Autodesk Inventor part; units mm, degrees
ref_plane "YZ Plane" through (0, 0, 0) normal (1, 0, 0) x (0, 1, 0)
ref_plane "XZ Plane" through (0, 0, 0) normal (0, 1, 0) x (-1, 0, 0)
ref_plane "XY Plane" through (0, 0, 0) normal (0, 0, 1) x (1, 0, 0)
sketch "Base" plane through (0, 0, 0) normal (0, 0, 1) x (1, 0, 0)
  line L0 (-22, -39.56) -> (22, -39.56)
  line L1 (22, -39.56) -> (22, 39.56)
  line L2 (22, 39.56) -> (-22, 39.56)
  line L3 (-22, 39.56) -> (-22, -39.56)
  line L4 (-22, -39.56) -> (22, 39.56) construction
  line L5 (22, -39.56) -> (-22, 39.56) construction
  point P0 (0, 0)
  dimension "d56" = 44
  dimension "d57" = 79.12
extrude "Extrusion4" add sketch "Base" along normal blind 6
sketch "Slot1" plane through (0, 0, 6) normal (0, 0, 1) x (1, 0, 0)
  line L0 (21, -38.56) -> (-21, -38.56)
  line L1 (-21, -38.56) -> (-21, -30.44)
  line L2 (-21, -30.44) -> (21, -30.44)
  line L3 (21, -30.44) -> (21, -38.56)
  line L4 (21, -38.56) -> (-21, -30.44) construction
  line L5 (-21, -38.56) -> (21, -30.44) construction
  line L6 (22, -39.56) -> (22, 39.56)
  line L7 (-22, -39.56) -> (22, -39.56)
  point P0 (0, 0)
  point P1 (0, -34.5)
  dimension "d62" = 8.12
  dimension "d63" = 1
  dimension "d64" = 42
  dimension "d66" = 1
extrude "Slot1 slot" cut sketch "Slot1" against normal blind 4
sketch "Slot2" plane through (0, 0, 6) normal (0, 0, 1) x (1, 0, 0)
  line L0 (21, -0.44) -> (-21, -0.44)
  line L1 (-21, -0.44) -> (-21, 6.08)
  line L2 (-21, 6.08) -> (21, 6.08)
  line L3 (21, 6.08) -> (21, -0.44)
  line L4 (21, -0.44) -> (-21, 6.08) construction
  line L5 (-21, -0.44) -> (21, 6.08) construction
  line L6 (-22, 39.56) -> (-22, -39.56)
  line L7 (-21, -30.44) -> (21, -30.44)
  point P0 (0, 0)
  point P1 (0, 2.82)
  dimension "d75" = 6.52
  dimension "d76" = 42
  dimension "d77" = 1
  dimension "d80" = 30
extrude "Slot2 slot" cut sketch "Slot2" against normal blind 4
sketch "Slot3" plane through (0, 0, 6) normal (0, 0, 1) x (1, 0, 0)
  line L0 (-21, 38.2) -> (21, 38.2)
  line L1 (21, 38.2) -> (21, 34.08)
  line L2 (21, 34.08) -> (-21, 34.08)
  line L3 (-21, 34.08) -> (-21, 38.2)
  line L4 (-21, 38.2) -> (21, 34.08) construction
  line L5 (21, 38.2) -> (-21, 34.08) construction
  point P0 (0, 36.14)
  dimension "d83" = 4.12
  dimension "d84" = 42
extrude "Extrusion7" cut sketch "Slot3" against normal blind 4
fillet "Fillet1" radius 2 1 edges at (-22, 39.56, 3)
fillet "Fillet2" radius 2 1 edges at (22, 39.56, 3)
fillet "Fillet3" radius 2 1 edges at (22, -39.56, 3)
fillet "Fillet4" radius 2 1 edges at (-22, -39.56, 3)
sketch "Sketch14" plane through (0, 0, 6) normal (0, 0, 1) x (1, 0, 0)
  point P0 (0, 0)
equation "\"d56\" = basew"
equation "\"d57\" = baseh"
equation "\"d62\" = wall1slot"
equation "\"d63\" = -0.5 * wallw + 0.5 * basew"
equation "\"d64\" = wallw"
equation "\"d66\" = 0.5 * baseextra"
equation "\"d75\" = wall2slot"
equation "\"d76\" = wallw"
equation "\"d77\" = 0.5 * baseextra"
equation "\"d80\" = gap1"
equation "\"d83\" = wall3slot"
equation "\"d84\" = wallw"
equation "\"printer3dtolerance\" = 0.12"
equation "\"wallw\" = 42"
equation "\"wallh\" = 44"
equation "\"cornerrad\" = 2"
equation "\"baseextra\" = 2"
equation "\"wall1_thick\" = 8"
equation "\"wall2_thick\" = 6.4"
equation "\"wall3_thick\" = 4"
equation "\"wall1slot\" = 8.12"
equation "\"wall2slot\" = 6.52"
equation "\"wall3slot\" = 4.12"
equation "\"gap1\" = 30"
equation "\"gap2\" = 28"
equation "\"baseh\" = 79.12"
equation "\"basew\" = 44"
equation "\"base_thick\" = 6"
equation "\"base_slots_depth\" = 4"
equation "\"d26\" = 8.12"
equation "\"d27\" = 42"
equation "\"d28\" = 44"
equation "\"d29\" = 28"
equation "\"d31\" = 4.12"
equation "\"d32\" = 6.52"
equation "\"d33\" = 79.12"
equation "\"d39\" = 8.12"
equation "\"d40\" = 42"
equation "\"d41\" = 44"
equation "\"d48\" = 8.12"
equation "\"d49\" = 42"
equation "\"d50\" = 8.12"
equation "\"d51\" = 42"
equation "\"d52\" = 44"
equation "\"d53\" = 44"
equation "\"d71\" = 8.12"
equation "\"d72\" = 42"
equation "\"d73\" = 2"
equation "\"d74\" = 44"
equation "\"distancefrombottom\" = 34"
equation "\"servosmallcircledia\" = 5.92"
equation "\"servo9gw\" = 22.8"
equation "\"servomountsquare\" = 6"
equation "\"servopolygonl\" = 5.92"
equation "\"servopolygonr\" = 6.12"
equation "\"distancefromleft\" = 26"
equation "\"servobigcircledia\" = 11.62"
equation "\"servomounth\" = 4"
equation "\"wall3slotd\" = 2"
equation "\"wall3slotw\" = 36"
equation "\"adapterh\" = 16"
equation "\"adapterw\" = 32"
equation "\"wall3slotd_1\" = 2"
properties part number "base-frame" material "Wood (Oak)"
Input: part model. Units: mm. Frame: model coordinates. A direction names the side the tool comes from. Coordinates: 2 decimals unless noted, no trailing zeros. Loops run counter-clockwise (first coordinate to the right, second up) from the corner with the lowest first, then second, coordinate; pieces in that order, holes last.
Q1. Contact query for a flat-ended pin moving along its axis: pin 1 (3.5 mm diameter, centred on x = -2, y = 1.5, fed in from +Z). Output: stop coordinate, or through.
Results are:
pin 1: stops at z = 2
Q2. Section B-B, the plane x = -3.5. Return the cut outline in (y, z).
Results are:
outline: (-39.56, 0) - (39.56, 0) - (39.56, 6) - (38.2, 6) - (38.2, 2) - (34.08, 2) - (34.08, 6) - (6.08, 6) - (6.08, 2) - (-0.44, 2) - (-0.44, 6) - (-30.44, 6) - (-30.44, 2) - (-38.56, 2) - (-38.56, 6) - (-39.56, 6) - close
Q3. Mould query, pull axis X, two halves, no side actions, for faces 3 (the cylindrical face through (-21.43, -38.96, 3.04)), 4 (the flat face through (0, 9, 6)), 5 (the flat face through (21, 36, 4)). Classes: +X half, -X half, draft (parallel to the pull), parting line (faces both ways), or undercut.
Results are:
face 3: -X half
face 4: draft
face 5: undercut
Q4. Section A-A, the plane z = 5.25. Return the cut outline in (x, y).
Results are:
outline: (-22, -37.56) arc R2 ccw to (-20, -39.56) - (20, -39.56) arc R2 ccw to (22, -37.56) - (22, 37.56) arc R2 ccw to (20, 39.56) - (-20, 39.56) arc R2 ccw to (-22, 37.56) - close; hole (-21, -38.56) - (21, -38.56) - (21, -30.44) - (-21, -30.44) - close; hole (-21, -0.44) - (21, -0.44) - (21, 6.08) - (-21, 6.08) - close; hole (-21, 34.08) - (21, 34.08) - (21, 38.2) - (-21, 38.2) - close
Q5. Line query: line 1 along Y through (x, z) = (-2, 2.65); line 2 along X through (y, z) = (-32, 4.45); line 3 along Z through (x, y) = (3, 0.5). Output: solid intervals per line, ascending.
Results are:
line 1: y = -39.56 to -38.56, -30.44 to -0.44, 6.08 to 34.08, 38.2 to 39.56
line 2: x = -22 to -21, 21 to 22
line 3: z = 0 to 2
Q6. Set-up query: faces 1 (the flat face through (22, -1, 3)), 2 (the flat face through (21, 3, 4)). Return all of +Z, -Z, +X, -X, +Y, -Y with unobstructed straight access to the full face (end or side cutting, diameter ignored); none if empty.
Results are:
face 1: +Z, -Z, +X, +Y, -Y
face 2: +Z
